```python
from build123d import *

# Parameters (mm, degrees)
SKETCH1_W             = 38.1
SKETCH1_H             = 44.45
BOSS_EXTRUDE1_DEPTH   = 3.175
F_6_CLEARANCE_HOLE1_D = 3.5052
CUT_EXTRUDE3_REACH    = 60.887
SKETCH6_W             = 12.7
SKETCH6_H             = 6.35
CUT_EXTRUDE4_REACH    = 60.887
SKETCH7_R             = 6
M3_CLEARANCE_HOLE1_D  = 3


with BuildPart() as part:
    # Sketch1 → Boss-Extrude1 (new, symmetric)
    with BuildSketch(Plane.XY):
        with Locations((19.05, -22.225)):
            Rectangle(SKETCH1_W, SKETCH1_H)
    extrude(amount=BOSS_EXTRUDE1_DEPTH, both=True)

    # #6 Clearance Hole1 (through all)
    with Locations(Plane.XY.offset(3.175)):
        with Locations((6.35, -3.175), (31.75, -3.175)):
            Hole(F_6_CLEARANCE_HOLE1_D / 2)

    # Sketch6 → Cut-Extrude3 (cut, up to next)
    with BuildSketch(Plane.XY.offset(3.175), mode=Mode.PRIVATE) as cut_extrude3_sk1:
        with Locations((19.05, -3.175)):
            Rectangle(SKETCH6_W, SKETCH6_H)
    cut_extrude3_tool1 = extrude(cut_extrude3_sk1.sketch, amount=-CUT_EXTRUDE3_REACH, mode=Mode.PRIVATE) & part.part
    add(cut_extrude3_tool1.solids().sort_by_distance((19.05, -3.175, 3.175))[0], mode=Mode.SUBTRACT)

    # Sketch7 → Cut-Extrude4 (cut, up to next)
    with BuildSketch(Plane.XY.offset(3.175), mode=Mode.PRIVATE) as cut_extrude4_sk1:
        with Locations((18.7325, -22.225)):
            Circle(SKETCH7_R)
    cut_extrude4_tool1 = extrude(cut_extrude4_sk1.sketch, amount=-CUT_EXTRUDE4_REACH, mode=Mode.PRIVATE) & part.part
    add(cut_extrude4_tool1.solids().sort_by_distance((18.7325, -22.225, 3.175))[0], mode=Mode.SUBTRACT)

    # M3 Clearance Hole1 (through all)
    with Locations(Plane.XY.offset(3.175)):
        with Locations((27.7325, -22.225), (9.7325, -22.225)):
            Hole(M3_CLEARANCE_HOLE1_D / 2)


solid = part.part
```
For this review, take the finished solid that the model builds, in its own axes (mm). A direction names the side the tool comes from. Round coordinates to 2 decimals unless told otherwise and drop trailing zeros. Loops run counter-clockwise (first coordinate to the right, second up) from the corner with the lowest first, then second, coordinate; pieces in that order, holes last.
Q1. Insertion check: pin 1 Ø3 at (x, z) = (21.5, 0.5) entering from +Y. The pin has a flat end and moves straight along its axis. Give the tip position at first contact, or say it passes through.
Result sheet:
pin 1: stops at y = -6.35
Q2. Mouldability with a two-part tool opening along Y and no side actions: class faces 1 (the face through (32, 0, 0)), 2 (the face through (29.23, -22.16, -0.04)), 3 (the face through (19, -44.45, 0)) as +Y half, -Y half, draft (parallel to the pull), parting line (faces both ways), or undercut.
Result sheet:
face 1: +Y half
face 2: undercut
face 3: -Y half
Q3. Add section B-B on z = -1.75. Give the number of separate pieces and of enclosed holes in the cut face, plus the area to 3 significant figures.
Result sheet:
separate pieces: 1
enclosed holes: 5
area: 1,470 mm2
Q4. Machinability: for faces 4 (the face through (12.7, -3, 0)), 5 (the face through (12.74, -21.96, 0.04)), which of the approach directions +Z, -Z, +X, -X, +Y, -Y give a long, thin tool a straight path to every point of the face, cutting with its end or side? Answer none if there is none.
Result sheet:
face 4: +Z, -Z, +Y
face 5: +Z, -Z
Q5. To check wall thickness, follow line 1 along X through (y, z) = (-3.5, 1.25); line 2 along X through (y, z) = (-23.5, -0.75); line 3 along Y through (x, z) = (31.75, -1.25). State the ranges of each line that lie inside material, in increasing order.
Result sheet:
line 1: x = 0 to 4.63, 8.07 to 12.7, 25.4 to 30.03, 33.47 to 38.1
line 2: x = 0 to 8.94, 10.52 to 12.87, 24.6 to 26.94, 28.52 to 38.1
line 3: y = -44.45 to -4.93, -1.42 to 0
Q6. Add section A-A on x = 31.75. Write out the cut boundary in (y, z) (3 decimals).
Result sheet:
outline: (-44.45, -3.175) - (-4.928, -3.175) - (-4.928, 3.175) - (-44.45, 3.175) - close; (-1.422, -3.175) - (0, -3.175) - (0, 3.175) - (-1.422, 3.175) - close
